Input: part model. Units: mm. Frame: model coordinates. A direction names the side the tool comes from. Coordinates: 2 decimals unless noted, no trailing zeros. Loops run counter-clockwise (first coordinate to the right, second up) from the corner with the lowest first, then second, coordinate; pieces in that order, holes last. Notation, with made-up numbers: (-12.75, 18) - (-8.75, 18) arc R24 cw to (-8.75, 43) - close; hole circle Ø9 at (76, -26). An arc over 180 degrees is marked (long way). Use one line per item in the form item = value.
from build123d import *

# Parameters (mm, degrees)
SKETCH1_R           = 7.747
SKETCH1_R_2         = 2.75
BOSS_EXTRUDE1_DEPTH = 1.65
BOSS_EXTRUDE3_START = 3.175
SKETCH2_W           = 15.24
SKETCH2_H           = 10.22657696
SKETCH2_R           = 2.75
BOSS_EXTRUDE3_DEPTH = 3.175


with BuildPart() as part:
    # Sketch1 → Boss-Extrude1 (new body)
    with BuildSketch(Plane.XY):
        with BuildLine():
            Line((43.669801091, 23.910175431), (31.75, 12.722643302))
            Line((31.75, 12.722643302), (31.75, 6.372643302))
            Line((31.75, 6.372643302), (43.669801091, -4.814888828))
            ThreePointArc((43.669801091, -4.814888828), (49.901216852, -8.767739159), (57.15, -10.150023865))
            ThreePointArc((57.15, -10.150023865), (64.398783148, -8.767739159), (70.630198909, -4.814888828))
            Line((70.630198909, -4.814888828), (82.55, 6.372643302))
            Line((82.55, 6.372643302), (82.55, 12.722643302))
            Line((82.55, 12.722643302), (70.630198909, 23.910175431))
            ThreePointArc((70.630198909, 23.910175431), (57.15, 29.245310468), (43.669801091, 23.910175431))
        make_face()
        with BuildLine():
            ThreePointArc((57.15, -1.424690282), (59.9, -4.174690282), (57.15, -6.924690282))
            ThreePointArc((57.15, -6.924690282), (54.4, -4.174690282), (57.15, -1.424690282))
        make_face(mode=Mode.SUBTRACT)
        with Locations(Location((57.15, 9.547643302, 0), (0, 0, 180))):
            Circle(SKETCH1_R, mode=Mode.SUBTRACT)
        with Locations(Location((57.15, 23.269976885, 0), (0, 0, 180))):
            Circle(SKETCH1_R_2, mode=Mode.SUBTRACT)
    extrude(amount=BOSS_EXTRUDE1_DEPTH)

    # Sketch2 → Boss-Extrude3 (add)
    # profile 1 of 2: a face of its own
    with BuildSketch(Plane(origin=(0, 0, 0), x_dir=(-1, 0, 0), z_dir=(0, 0, -1)).offset(BOSS_EXTRUDE3_START)):
        with Locations((-57.15, 22.598431782)):
            Rectangle(SKETCH2_W, SKETCH2_H)
        with Locations((-57.15, 23.269976885)):
            Circle(SKETCH2_R, mode=Mode.SUBTRACT)
    # profile 2 of 2: a face of its own
    with BuildSketch(Plane(origin=(0, 0, 0), x_dir=(-1, 0, 0), z_dir=(0, 0, -1)).offset(BOSS_EXTRUDE3_START)):
        with Locations((-57.15, -3.503145178)):
            Rectangle(SKETCH2_W, SKETCH2_H)
        with Locations((-57.15, -4.174690282)):
            Circle(SKETCH2_R, mode=Mode.SUBTRACT)
    extrude(amount=-BOSS_EXTRUDE3_DEPTH)


solid = part.part
Q1. Set-up query: faces 5 (the flat face through (57, 28, 0)), 6 (the flat face through (57, -9, 0)), 7 (the flat face through (49.53, 23, -2)), 8 (the flat face through (64.77, 23, -2)). Return all of +Z, -Z, +X, -X, +Y, -Y with unobstructed straight access to the full face (end or side cutting, diameter ignored); none if empty.
Check values:
face_5 = -Z, +X, -X, +Y
face_6 = -Z, +X, -X, -Y
face_7 = -Z, -X, +Y, -Y
face_8 = -Z, +X, +Y, -Y
Q2. Cut plane C-C, the plane z = -2.5. Return loops of the section in (x, y), then the cut area to 3 significant figures.
Check values:
outline = (49.53, -8.62) - (64.77, -8.62) - (64.77, 1.61) - (49.53, 1.61) - close; (49.53, 17.49) - (64.77, 17.49) - (64.77, 27.71) - (49.53, 27.71) - close; hole circle Ø5.5 at (57.15, -4.17); hole circle Ø5.5 at (57.15, 23.27)
area = 264 mm²
Q3. Cut plane A-A, the plane y = 11.5. Return loops of the section in (x, z), then the cut area to 3 significant figures.
Check values:
outline = (31.75, 0) - (49.65, 0) - (49.65, 1.65) - (31.75, 1.65) - close; (64.65, 0) - (82.55, 0) - (82.55, 1.65) - (64.65, 1.65) - close
area = 59.1 mm²
Q4. First-contact query: P1, Ø12, axis at x = 45.5, y = 11.5, coming from the -Z side; P2, Ø2.5, axis at y = -2, z = -1.5, coming from the +X side; P3, Ø2.5, axis at y = 23, z = -1.5, coming from the -X side. Flat tips, straight axial feed; report the tip coordinate or a pass-through.
Check values:
P1 = 0
P2 = 64.77
P3 = 49.53
Q5. Cut plane B-B, the plane x = 64. Return loops of the section in (y, z) (3 decimals).
Check values:
outline = (-8.921, 0) - (-8.616, 0) - (-8.616, -3.175) - (1.61, -3.175) - (1.61, 0) - (5.929, 0) - (5.929, 1.65) - (-8.921, 1.65) - close; (13.166, 0) - (17.485, 0) - (17.485, -3.175) - (27.712, -3.175) - (27.712, 0) - (28.016, 0) - (28.016, 1.65) - (13.166, 1.65) - close
Q6. Cut plane D-D, the plane z = 1.05. Return loops of the section in (x, y), then the cut area to 3 significant figures.
Check values:
outline = (31.75, 6.37) - (43.67, -4.81) arc R19.7 ccw to (70.63, -4.81) - (82.55, 6.37) - (82.55, 12.72) - (70.63, 23.91) arc R19.7 ccw to (43.67, 23.91) - (31.75, 12.72) - close; hole circle Ø15.49 at (57.15, 9.55); hole circle Ø5.5 at (57.15, -4.17); hole circle Ø5.5 at (57.15, 23.27)
area = 1,150 mm²
Q7. Ray query, line 1 along Y through (x, z) = (57.15, 0.6); line 2 along Y through (x, z) = (57, -1.85); line 3 along Y through (x, z) = (63, -0.3). Return the intervals inside material, ascending. Write a range as [from, to].
Check values:
line_1 = [-10.15, -6.92], [-1.42, 1.8], [17.29, 20.52], [26.02, 29.25]
line_2 = [-8.62, -6.92], [-1.43, 1.61], [17.49, 20.52], [26.02, 27.71]
line_3 = [-8.62, 1.61], [17.49, 27.71]
Q8. Pull-direction query (Y, two-part tool) for faces 1 (the cylindrical face through (57.358, 29.244, 0.813)), 2 (the flat face through (76.507, 0.701, 0.813)), 3 (the flat face through (57, 1.61, -2)), 4 (the flat face through (57, 17.485, -2)); classes: pulls with the +Y half, pulls with the -Y half, needs draft (parallel to the pull), parting line crosses it, or undercut.
Check values:
face_1 = pulls with the +Y half
face_2 = pulls with the -Y half
face_3 = undercut
face_4 = undercut
